Part model, mm, in its own coordinate system. A direction names the side the tool comes from. Coordinates: 2 decimals unless noted, no trailing zeros. Loops run counter-clockwise (first coordinate to the right, second up) from the corner with the lowest first, then second, coordinate; pieces in that order, holes last. Notation, with made-up numbers: (-33, 7) -> (-25, 7) arc R24 ccw to (-25, 36) -> close; hole circle Ø7 at (64, -1.75). An arc over 180 degrees is marked (long way). One line per question, with ' | ' between items. Start each with the question number.
1) 3-axis set-ups, long thin cutter, end or side, ignore diameter. For faces 1 (the face through (3, 0, 1.8)), 2 (the face through (-5.158, -3.955, 0.887)): which of +Z, -Z, +X, -X, +Y, -Y reach the whole face in a straight line?
2) Cut at C-C (z = 3). List the corners of the cut face in (x, y), plus the area to 3 significant figures.
3) Cut at A-A (x = 0). List the corners of the cut face in (y, z), plus the area to 3 significant figures.
4) Probe L1, parallel to Z at x = -2, y = -2.5; L2, parallel to Z at x = -4.5, y = 2; L3, parallel to Z at x = -3, y = -2.75. List the from-to ranges inside material, lowest first. Write a range as from..to.
5) Cut at D-D (z = 11). List the corners of the cut face in (x, y).
6) Drop flat-ended pins along their axis: pin 1 (2 mm diameter, centred on x = 0.5, y = 1, fed in from +Z); pin 2 (5 mm diameter, centred on x = 2, z = 7.5, fed in from -Y); pin 3 (1.5 mm diameter, centred on x = 0.5, z = 10.5, fed in from -Y). Give the stop position or say it passes through.
7) Two-plate mould, pull along Z, no slides. Class faces 3 (the face through (-0.27, -1.22, 7.05)), 4 (the face through (0, 0, 0)), 5 (the face through (4.197, 1.322, 4.794)): released by +Z, released by -Z, zero draft, split by the parting line, or undercut.
from build123d import *

# Parameters (mm, degrees)
F0_R     = 6.5
F1_DEPTH = 1.8
F2_R     = 2.6
F4_DEPTH = 2.6
F5_R     = 4.4
F6_DEPTH = 1.8
F7_SIZE  = 1
F8_R     = 1.25
F9_DEPTH = 1.8


with BuildPart() as f1:
    # F0 (on Top) → F1 (new body)
    with BuildSketch(Plane.XY):
        Circle(F0_R)
    extrude(amount=F1_DEPTH)

    # F2 (on face) → F4 (join)
    with BuildSketch(Plane.XY.offset(1.8)):
        Circle(F2_R)
    extrude(amount=F4_DEPTH)

    # F5 (on face) → F6 (join, through all)
    with BuildSketch(Plane.XY.offset(4.4)):
        Circle(F5_R)
    extrude(amount=F6_DEPTH)

    # F7
    f7_edges = [f1.edges().sort_by_distance(p)[0] for p in [
        (-4.4, 0, 6.2),
    ]]
    chamfer(f7_edges, length=F7_SIZE)

    # F8 (on face) → F9 (join)
    with BuildSketch(Plane.XY.offset(6.2)):
        Circle(F8_R)
    extrude(amount=F9_DEPTH)

    # F10 (on Right) → F11 (revolve)
    with BuildSketch(Plane.YZ):
        with BuildLine():
            Line((0, 12.05), (0, 7.55))
            ThreePointArc((0, 7.55), (2.25, 9.8), (0, 12.05))
        make_face()
    revolve(axis=Axis((0, 0, 9.8), (0, 0, 1)))


solid = f1.part
Reported:
1) face 1: none | face 2: +Z, -Z
2) outline: circle Ø5.2 at (0, 0) | area: 21.2 mm²
3) outline: (-6.5, 0) -> (6.5, 0) -> (6.5, 1.8) -> (2.6, 1.8) -> (2.6, 4.4) -> (4.4, 4.4) -> (4.4, 5.2) -> (3.4, 6.2) -> (1.25, 6.2) -> (1.25, 7.93) arc R2.25 ccw (long way) to (-1.25, 7.93) -> (-1.25, 6.2) -> (-3.4, 6.2) -> (-4.4, 5.2) -> (-4.4, 4.4) -> (-2.6, 4.4) -> (-2.6, 1.8) -> (-6.5, 1.8) -> close | area: 71.3 mm²
4) L1: z = 0..1.8, 4.4..6.2 | L2: z = 0..1.8 | L3: z = 0..1.8, 4.4..5.53
5) outline: circle Ø3.81 at (0, 0)
6) pin 1: stops at z = 12.05 | pin 2: stops at y = -4.28 | pin 3: stops at y = -2.25
7) face 3: undercut | face 4: released by -Z | face 5: zero draft
